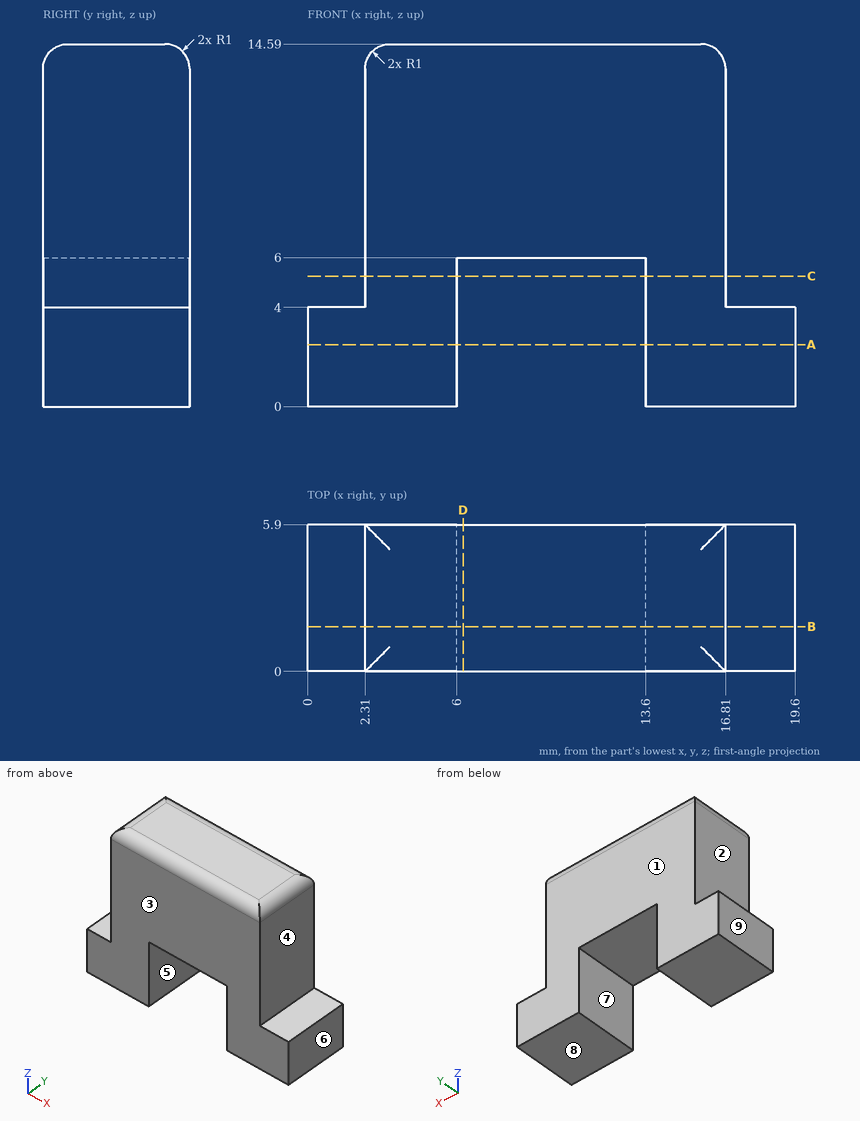
Verification items for this drawing (mm, ordinates from the low corner). A direction names the side the tool comes from. Coordinates: 2 decimals unless noted, no trailing zeros. Loops run counter-clockwise (first coordinate to the right, second up) from the corner with the lowest first, then second, coordinate; pieces in that order, holes last.
Item 1: Thickness scan on line 1 (X direction, y = 3.05, z = 1.25); line 2 (Z direction, x = 1.75, y = 5); line 3 (X direction, y = 5.5, z = 5.25). Record the ranges inside material, lowest first.
Item 2: Sectioned sample at B-B, the plane y = 1.8. Record the boundary of the cut face in (x, z).
Item 3: Release check for a two-part mould opening along X. For the marked faces 6, 7, 8 and 9 record: released by +X, released by -X, zero draft, split by the parting line, or undercut.
Item 4: Access from +Z, -Z, +X, -X, +Y, -Y to the whole of each face (thin tool, end or side, straight path). Record for the marked faces 1, 2, 3, 4 and 5.
Item 5: Sectioned sample at D-D, the plane x = 6.25. Record the boundary of the cut face in (y, z).
Item 6: Go/stop test with flat-tipped pins: pin 1 Ø2 at (x, y) = (12.5, 5.5) entering from -Z; pin 2 Ø1.8 at (y, z) = (3, 8.5) entering from -X; pin 3 Ø1.2 at (x, y) = (1.5, 2.5) entering from +Z. Record where each tip stops, or that it passes through.
Item 7: Sectioned sample at A-A, the plane z = 2.5. Record the boundary of the cut face in (x, y).
Item 8: Sectioned sample at C-C, the plane z = 5.25. Record the boundary of the cut face in (x, y).
Check result:
1. line 1: x = 0 to 6, 13.6 to 19.6
1. line 2: z = 0 to 4
1. line 3: x = 2.31 to 6, 13.6 to 16.81
2. outline: (0, 0) - (6, 0) - (6, 6) - (13.6, 6) - (13.6, 0) - (19.6, 0) - (19.6, 4) - (16.81, 4) - (16.81, 13.59) arc R1 ccw to (15.81, 14.59) - (3.31, 14.59) arc R1 ccw to (2.31, 13.59) - (2.31, 4) - (0, 4) - close
3. face 6: released by +X
3. face 7: undercut
3. face 8: zero draft
3. face 9: released by -X
4. face 1: +Z, -Z, +X, -X, +Y
4. face 2: +Z, -X, +Y, -Y
4. face 3: +Z, -Z, +X, -X, -Y
4. face 4: +Z, +X, +Y, -Y
4. face 5: -Z, +Y, -Y
5. outline: (0, 6) - (5.9, 6) - (5.9, 13.59) arc R1 ccw to (4.9, 14.59) - (1, 14.59) arc R1 ccw to (0, 13.59) - close
6. pin 1: stops at z = 6
6. pin 2: stops at x = 2.31
6. pin 3: stops at z = 4
7. outline: (0, 0) - (6, 0) - (6, 5.9) - (0, 5.9) - close; (13.6, 0) - (19.6, 0) - (19.6, 5.9) - (13.6, 5.9) - close
8. outline: (2.31, 0) - (6, 0) - (6, 5.9) - (2.31, 5.9) - close; (13.6, 0) - (16.81, 0) - (16.81, 5.9) - (13.6, 5.9) - close
